Check sheet for the drawn part. Datum: minimum x, y, z corner. Units: mm. A direction names the side the tool comes from. Coordinates: 2 decimals unless noted, no trailing zeros. Loops run counter-clockwise (first coordinate to the right, second up) from the corner with the lowest first, then second, coordinate; pieces in that order, holes last. Notation, with made-up numbers: (-17, 33.25) -> (39, 33.25) arc R23 ccw to (39, 50.25) -> close; hole circle Ø4 at (20.5, 23.5). An arc over 180 degrees is marked (long way). Use CSV: the item, a comma, the result in double quotes. Start each with the question number.
1. Gauge pin test, flat ends, axial feed: pin 1 (3 mm diameter, centred on x = 16, z = 18, fed in from -Y); pin 2 (7.5 mm diameter, centred on x = 27, y = 9.5, fed in from +Z); pin 3 (10 mm diameter, centred on x = 5.5, z = 21, fed in from -Y); pin 4 (8 mm diameter, centred on y = 18, z = 15, fed in from +X). Record the tip position at first contact, or that the pin passes through.
2. Sectioned sample at C-C, the plane z = 9.75. Record the cut outline in (x, y).
3. Sectioned sample at B-B, the plane y = 19.75. Record the cut outline in (x, z).
4. Thickness scan on L1, parallel to X at y = 20.5, z = 17.5; L2, parallel to Z at x = 31, y = 10.5; L3, parallel to Z at x = 5, y = 6.5 (1 decimal). Record the ranges inside material, lowest first.
5. Sectioned sample at A-A, the plane x = 2.5. Record the cut outline in (y, z), and give its area (3 significant figures).
6. Sectioned sample at D-D, the plane x = 33.5. Record the cut outline in (y, z), and give its area (3 significant figures).
7. Set-up check for the marked faces 1 and 2: record each of +Z, -Z, +X, -X, +Y, -Y from which the full face is reachable in a straight line by a thin tool's end or side.
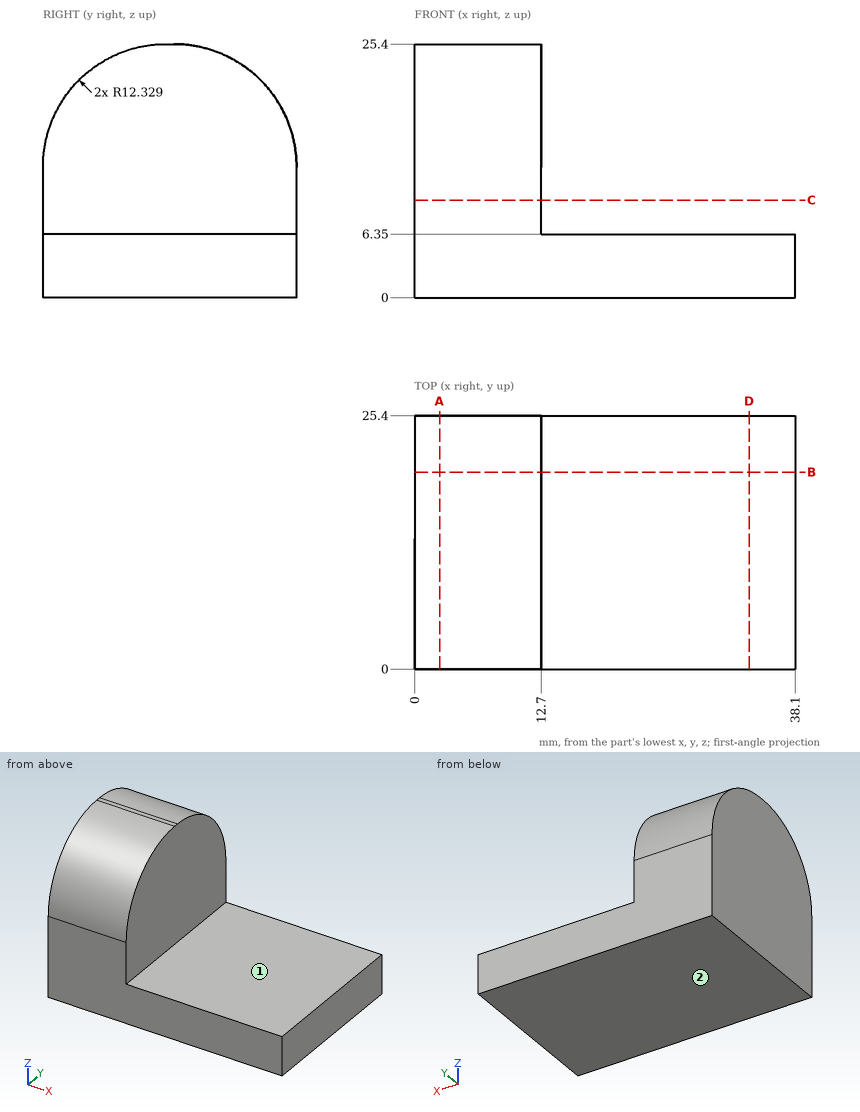
Completed:
1,pin 1,"through"
1,pin 2,"z = 6.35"
1,pin 3,"y = 0.35"
1,pin 4,"x = 12.7"
2,outline,"(0, 0) -> (12.7, 0) -> (12.7, 25.4) -> (0, 25.4) -> close"
3,outline,"(0, 0) -> (38.1, 0) -> (38.1, 6.35) -> (12.7, 6.35) -> (12.7, 23.43) -> (0, 23.43) -> close"
4,L1,"0 to 12.7"
4,L2,"0 to 6.35"
4,L3,"0 to 23.9"
5,outline,"(0, 0) -> (25.4, 0) -> (25.4, 13.07) arc R12.33 ccw to (13.07, 25.4) -> (12.33, 25.4) arc R12.33 ccw to (0, 13.07) -> close"
5,area,"580 mm²"
6,outline,"(0, 0) -> (25.4, 0) -> (25.4, 6.35) -> (0, 6.35) -> close"
6,area,"161 mm²"
7,face 1,"+Z, +X, +Y, -Y"
7,face 2,"-Z, +X, -X, +Y, -Y"
